```python
from build123d import *

# Parameters (mm, degrees)
SKETCH_R      = 12.5
SKETCH_R_2    = 1.7
SKETCH_R_3    = 4.15
PAD_DEPTH     = 5
SKETCH001_R   = 6.5
SKETCH001_R_2 = 4.05
PAD001_DEPTH  = 5


with BuildPart() as part:
    # Sketch → Pad (new body)
    with BuildSketch(Plane.XY):
        Circle(SKETCH_R)
        with Locations((0, 9.5)):
            Circle(SKETCH_R_2, mode=Mode.SUBTRACT)
        with Locations((-9.5, 0)):
            Circle(SKETCH_R_2, mode=Mode.SUBTRACT)
        with Locations((0, -9.5)):
            Circle(SKETCH_R_2, mode=Mode.SUBTRACT)
        with Locations((9.5, 0)):
            Circle(SKETCH_R_2, mode=Mode.SUBTRACT)
        Circle(SKETCH_R_3, mode=Mode.SUBTRACT)
    extrude(amount=PAD_DEPTH)

    # Sketch001 → Pad001 (join)
    with BuildSketch(Plane.XY.offset(5)):
        Circle(SKETCH001_R)
        Circle(SKETCH001_R_2, mode=Mode.SUBTRACT)
    extrude(amount=PAD001_DEPTH)


solid = part.part
```
Read the model definition and answer for the solid it produces. Units are mm, in the model's axes. A direction names the side the tool comes from. Coordinates: 2 decimals unless noted, no trailing zeros. Loops run counter-clockwise (first coordinate to the right, second up) from the corner with the lowest first, then second, coordinate; pieces in that order, holes last. Notation, with made-up numbers: (-14.75, -14.75) -> (40.25, -14.75) arc R20 ccw to (40.25, -9.75) -> close; hole circle Ø5 at (72.5, 68). An arc over 180 degrees is marked (long way). Return JSON: item names as keys, results as strings.
Item 1: For faces 1 (the cylindrical face through (-0.878, -3.954, 7.465)), 2 (the cylindrical face through (-0.9, -4.05, 2.46)), determine the directions among +Z, -Z, +X, -X, +Y, -Y from which every point of the face is accessible in a straight line to the end or side of a thin tool.
Answers:
{"face 1": "+Z, -Z", "face 2": "-Z"}
Item 2: Find section A-A (y = 0). Determine the outline of the cut face in (x, z), plus the area to 3 significant figures.
Answers:
{"outline": "(-12.5, 0) -> (-11.2, 0) -> (-11.2, 5) -> (-12.5, 5) -> close; (-7.8, 0) -> (-4.15, 0) -> (-4.15, 5) -> (-4.05, 5) -> (-4.05, 10) -> (-6.5, 10) -> (-6.5, 5) -> (-7.8, 5) -> close; (4.05, 5) -> (4.15, 5) -> (4.15, 0) -> (7.8, 0) -> (7.8, 5) -> (6.5, 5) -> (6.5, 10) -> (4.05, 10) -> close; (11.2, 0) -> (12.5, 0) -> (12.5, 5) -> (11.2, 5) -> close", "area": "74.0 mm2"}
Item 3: Find the intervals of material crossed by probe 1 along Y at (x, z) = (0, 1.1); probe 2 along Z at (x, y) = (-11, -1.25); probe 3 along Y at (x, z) = (9.5, 3.7), in increasing order.
Answers:
{"probe 1": "y = -12.5 to -11.2, -7.8 to -4.15, 4.15 to 7.8, 11.2 to 12.5", "probe 2": "z = 0 to 5", "probe 3": "y = -8.12 to -1.7, 1.7 to 8.12"}
Item 4: For a pull along X with two mould halves and no side action, classify faces 3 (the flat face through (5, -5, 5)), 4 (the cylindrical face through (-9.87, -1.66, 2.46)), 5 (the cylindrical face through (-5.158, -3.955, 7.465)), 6 (the cylindrical face through (8.15, -1.03, 2.46)) as +X half, -X half, draft (parallel to the pull), parting line (faces both ways), or undercut.
Answers:
{"face 3": "draft", "face 4": "undercut", "face 5": "parting line", "face 6": "undercut"}
Item 5: Find section D-D (x = 9.5). Determine the outline of the cut face in (y, z), plus the area to 3 significant figures.
Answers:
{"outline": "(-8.12, 0) -> (-1.7, 0) -> (-1.7, 5) -> (-8.12, 5) -> close; (1.7, 0) -> (8.12, 0) -> (8.12, 5) -> (1.7, 5) -> close", "area": "64.2 mm2"}
Item 6: Find section B-B (z = 2.75). Determine the outline of the cut face in (x, y).
Answers:
{"outline": "circle Ø25 at (0, 0); hole circle Ø3.4 at (-9.5, 0); hole circle Ø8.3 at (0, 0); hole circle Ø3.4 at (0, -9.5); hole circle Ø3.4 at (0, 9.5); hole circle Ø3.4 at (9.5, 0)"}
Item 7: Flat-ended cylindrical pins translate along their axes: P1, Ø1, axis at y = -8, z = 2.5, coming from the -X side; P2, Ø2, axis at y = 3.5, z = 6.5, coming from the +X side; P3, Ø6.5, axis at x = 0, y = 0, coming from the -Z side (1 decimal); P4, Ø5.5, axis at x = 0, y = -9.5, coming from the +Z side. Find the tip coordinate at first contact, or state that the pin passes through.
Answers:
{"P1": "stops at x = -10", "P2": "stops at x = 6", "P3": "passes through", "P4": "stops at z = 5"}
